Autodesk Fusion 360 part; units mm, degrees
sketch "Bracket Profile" plane through (0, 0, 0) normal (0, 0, 1) x (1, 0, 0) in component "Bracket"
  line L0 (0, 0) -> (0, 25)
  line L1 (0, 25) -> (5, 25)
  line L2 (5, 25) -> (5, 20)
  line L3 (5, 20) -> (5, 0)
  line L4 (5, 0) -> (0, 0)
  dimension "d1" = 5
  dimension "d2" = 5
  dimension "d3" = 25
  dimension "d4" = 5
extrude "Extrude1" add sketch "Bracket Profile" along normal blind 20 in component "Bracket"
sketch "Clearance Hole" plane through (0, 0, 0) normal (-1, 0, 0) x (0, -1, 0) in component "Bracket"
  line L0 (-25, 0) -> (0, 0)
  line L1 (0, 0) -> (0, 20)
  line L2 (0, 20) -> (-25, 20)
  line L3 (-25, 20) -> (-25, 0)
  line L4 (-25, 10) -> (0, 10) construction
  line L5 (-12.5, 20) -> (-12.5, 0) construction
  circle A0 centre (-12.5, 10) radius 2.9
  circle A1 centre (-12.5, 10) radius 4.5
  line L6 (0, 13) -> (-25, 13)
  line L7 (-25, 13) -> (-25, 7)
  line L8 (-25, 7) -> (0, 7)
  line L9 (0, 7) -> (0, 13)
  line L10 (0, 13) -> (-25, 7) construction
  line L11 (-25, 13) -> (0, 7) construction
  line L12 (-6.5, 13) -> (-18.5, 13)
  line L13 (-18.5, 13) -> (-18.5, 7)
  line L14 (-18.5, 7) -> (-6.5, 7)
  line L15 (-6.5, 7) -> (-6.5, 13)
  line L16 (-6.5, 13) -> (-18.5, 7) construction
  line L17 (-18.5, 13) -> (-6.5, 7) construction
  point P0 (-12.5, 10)
  point P1 (-12.5, 10)
  dimension "d9" = 5.8
  dimension "d13" = 9
  dimension "d20" = 25
  dimension "d21" = 6
  dimension "d24" = 12
  dimension "d25" = 6
extrude "Extrude3" add sketch "Clearance Hole" along normal blind 6 contours L3 L6 L7 L8 L13 | L1 L6 L8 L9 L15 in component "Bracket"
hole "Hole1" at (0, 12.5, 10) direction (1, 0, 0) diameter 5.8 end through all in component "Bracket"
sketch "Sketch3" plane through (0, 25, 0) normal (0, 1, 0) x (-1, 0, 0) in component "Bracket"
  line L0 (-5, 0) -> (0, 0)
  line L1 (0, 0) -> (0, 7)
  line L2 (0, 7) -> (6, 7)
  line L3 (6, 7) -> (6, 13)
  line L4 (6, 13) -> (0, 13)
  line L5 (0, 13) -> (0, 20)
  line L6 (0, 20) -> (-5, 20)
  line L7 (0, 20) -> (-25, 20)
  line L8 (-25, 20) -> (-25, 15)
  line L9 (-25, 15) -> (0, 15)
  line L10 (0, 15) -> (0, 20)
  line L11 (-5, 20) -> (-5, 0)
  dimension "d28" = 25
  dimension "d29" = 5
extrude "Extrude5" add 1 faces at (1.6667, 16.6667, 0) along direction (0, 0, -1) blind 5 in component "Bracket"
chamfer "Chamfer2" distance 0.8 angle 45 12 faces at (0, 12.5, -0.9667) (-6, 4.3333, 11) (-6, 22.8333, 11) (3.3333, 25, 7.3333) (1.6667, 16.6667, 20) (-2, 20.6667, 13) (-2, 2.1667, 13) (-2, 6.5, 9) (-4, 18.5, 9) (3.3333, 0, 7.3333) (5, 12.5, -0.9667) (1.6667, 16.6667, -5) in component "Bracket"
component "Bracket" placed x (1, 0, 0) y (0, 1, 0) z (0, 0, 1) at (0, 0, 0)
equation "d1 = BracketLipSize"
equation "d2 = BracketLipSize"
equation "d3 = ExtrusionSize + BracketLipSize"
equation "d4 = BracketLipSize"
equation "ExtrusionSize = 20 mm"
equation "BracketLipSize = 5 mm"
equation "d7 = ExtrusionSize"
equation "d9 = ScrewClearanceHole"
equation "ScrewClearanceHole = 5.8 mm"
equation "d11 = ScrewClearanceHole"
equation "d13 = ScrewHeadClearance"
equation "ScrewHeadClearance = 9 mm"
equation "Chamfer = 0.8 mm"
equation "Tounge = 6 mm"
equation "d20 = ExtrusionSize + BracketLipSize"
equation "d21 = Tounge"
equation "d22 = Tounge"
equation "d24 = NutClearance"
equation "d25 = Tounge"
equation "NutClearance = 12 mm"
equation "d28 = ExtrusionSize + BracketLipSize"
equation "d29 = BracketLipSize"
equation "d32 = BracketLipSize"
equation "d34 = Chamfer"
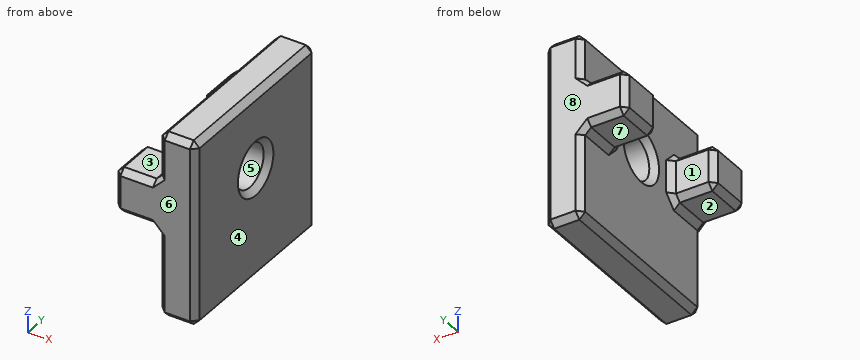
Can you work these out from the model? Positions are in its coordinate system, mm. Face numbers are marked on the shaded views. A direction names the side the tool comes from. Round coordinates to 2 decimals unless told otherwise and drop trailing zeros. Loops run counter-clockwise (first coordinate to the right, second up) from the corner with the lowest first, then second, coordinate; pieces in that order, holes last.
Item 1: Suppose I cut it at C-C, the plane z = 10. Write out the boundary of the cut face in (x, y), then the cut area to 3 significant figures.
Item 2: Suppose I cut it at A-A, the plane y = 12.5. Write out the boundary of the cut face in (x, z), then the cut area to 3 significant figures.
Item 3: If we mould it in two halves opening along Y, with no side actions, what happens to the marked faces 5, 6, 7 and 8? For each: +Y half, -Y half, draft (parallel to the pull), parting line (faces both ways), or undercut.
Item 4: Please list where these lines run through material, in increasing order: L1, parallel to Y at x = 2.8, z = 10; L2, parallel to Z at x = 2.15, y = 12.5; L3, parallel to Y at x = -3.75, z = 11.
Item 5: Suppose I cut it at B-B, the plane x = -4. Write out the boundary of the cut face in (y, z).
Item 6: Which directions (+Z, -Z, +X, -X, +Y, -Y) give clear straight access to the entire face, cutting with the end or side of a thin tool? Please do the marked faces 1, 2, 3 and 4.
Item 7: Will these pins go through, and if not, where does the flat tip stop? pin 1 Ø5 at (x, y) = (-4, 21.5) entering from +Z; pin 2 Ø7.5 at (y, z) = (12.5, 10) entering from -X; pin 3 Ø1 at (x, y) = (-1, 20.5) entering from -Z; pin 4 Ø2 at (x, z) = (-4, 10.5) entering from -Y.
Item 8: Suppose I cut it at D-D, the plane y = 2.75. Write out the boundary of the cut face in (x, z).
Reported:
1. outline: (-6, 0.8) - (-5.2, 0) - (4.2, 0) - (5, 0.8) - (5, 8.8) - (4.2, 9.6) - (0.8, 9.6) - (0, 8.8) - (0, 7.3) - (-0.8, 6.5) - (-5.2, 6.5) - (-6, 5.7) - close; (-6, 19.3) - (-5.2, 18.5) - (-0.8, 18.5) - (0, 17.7) - (0, 16.2) - (0.8, 15.4) - (4.2, 15.4) - (5, 16.2) - (5, 24.2) - (4.2, 25) - (-5.2, 25) - (-6, 24.2) - close
1. area: 171 mm2
2. outline: (0, -4.2) - (0.8, -5) - (4.2, -5) - (5, -4.2) - (5, 6.3) - (4.2, 7.1) - (0.8, 7.1) - (0, 6.3) - close; (0, 13.7) - (0.8, 12.9) - (4.2, 12.9) - (5, 13.7) - (5, 19.2) - (4.2, 20) - (0.8, 20) - (0, 19.2) - close
2. area: 93.4 mm2
3. face 5: undercut
3. face 6: -Y half
3. face 7: draft
3. face 8: +Y half
4. L1: y = 0 to 9.6, 15.4 to 25
4. L2: z = -5 to 7.1, 12.9 to 20
4. L3: y = 0 to 6.5, 18.5 to 25
5. outline: (0, 7.8) - (0.8, 7) - (5.7, 7) - (6.5, 7.8) - (6.5, 12.2) - (5.7, 13) - (0.8, 13) - (0, 12.2) - close; (18.5, 7.8) - (19.3, 7) - (24.2, 7) - (25, 7.8) - (25, 12.2) - (24.2, 13) - (19.3, 13) - (18.5, 12.2) - close
6. face 1: +Z, -Z, -X
6. face 2: -Z, -X, +Y, -Y
6. face 3: +Z, -X, +Y, -Y
6. face 4: +Z, -Z, +X, +Y, -Y
7. pin 1: stops at z = 13
7. pin 2: stops at x = 0
7. pin 3: stops at z = 6.7
7. pin 4: stops at y = 0
8. outline: (-6, 7.8) - (-5.2, 7) - (-0.8, 7) - (0, 6.2) - (0, -4.2) - (0.8, -5) - (4.2, -5) - (5, -4.2) - (5, 19.2) - (4.2, 20) - (0.8, 20) - (0, 19.2) - (0, 13.8) - (-0.8, 13) - (-5.2, 13) - (-6, 12.2) - close
